The model under review builds one solid part; all positions refer to its coordinate system, in mm. Face numbers are marked on the shaded views. A direction names the side the tool comes from. Give positions to 0.01 mm unless a question says otherwise; leave off trailing zeros. Loops run counter-clockwise (first coordinate to the right, second up) from the corner with the lowest first, then second, coordinate; pieces in that order, holes last. Notation, with made-up numbers: M -14.5,7 L 42.5,7 A20 ccw 42.5,32 Z; hole C 58.25,80 d10. An arc over 180 degrees is marked long. Return JSON: item names as keys, results as strings.
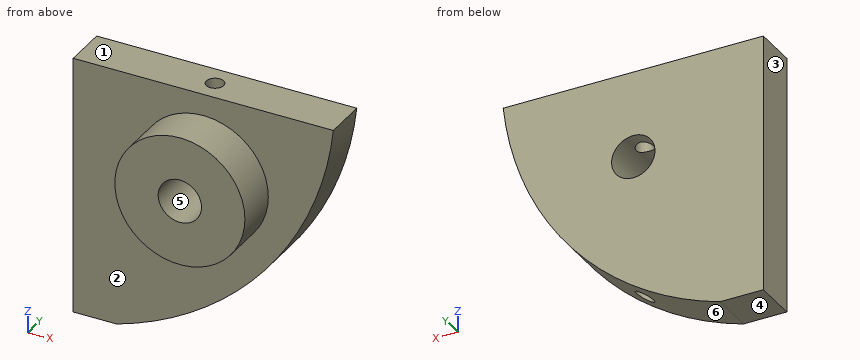
```python
from build123d import *

# Parameters (mm, degrees)
F1_DEPTH = 6.35
F2_R     = 19.05
F3_DEPTH = 12.7
F4_R     = 6.35
F5_DEPTH = 74.422
F6_R     = 2.54
F7_DEPTH = 76.201


with BuildPart() as f1:
    # F0 (on Front) → F1 (new body, symmetric)
    with BuildSketch(Plane.XZ):
        with BuildLine():
            Line((2.516038, 58.73151), (-73.683962, 58.73151))
            Line((-73.683962, 58.73151), (-73.683962, -17.46849))
            Line((-73.683962, -17.46849), (-60.983962, -17.46849))
            ThreePointArc((-60.983962, -17.46849), (-17.618712, 10.952135), (2.516038, 58.73151))
        make_face()
    extrude(amount=F1_DEPTH, both=True)

    # F2 (on face) → F3 (join)
    with BuildSketch(Plane.XZ.offset(6.35)):
        with Locations((-35.583962, 33.33151)):
            Circle(F2_R)
    extrude(amount=F3_DEPTH)

    # F4 (on face) → F5 (cut)
    with BuildSketch(Plane.XZ.offset(19.05)):
        with Locations((-35.583962, 33.33151)):
            Circle(F4_R)
    extrude(amount=-F5_DEPTH, mode=Mode.SUBTRACT)

    # F6 (on face) → F7 (cut, through all)
    with BuildSketch(Plane.XY.offset(58.73151)):
        with Locations((-35.583962, 0)):
            Circle(F6_R)
    extrude(amount=-F7_DEPTH, mode=Mode.SUBTRACT)


solid = f1.part
```
1) Consider section C-C on x = -50.5. Write out the cut boundary in (y, z), then the cut area to 3 significant figures.
From the geometry:
{"outline": "M -19.05,21.48 L -6.35,21.48 L -6.35,-13.68 L 6.35,-13.68 L 6.35,58.73 L -6.35,58.73 L -6.35,45.18 L -19.05,45.18 Z", "area": "1,220 mm²"}
2) Insertion check: pin 1 (6.5 mm diameter, centred on x = -35.58, y = 0, fed in from -Z); pin 2 (8 mm diameter, centred on x = -35.58, y = 0, fed in from -Z); pin 3 (8 mm diameter, centred on y = 2.5, z = 16, fed in from +X); pin 4 (4 mm diameter, centred on y = -7.5, z = 16, fed in from -X). Each pin has a flat end and moves straight along its axis. Give the tip position at first contact, or say it passes through.
From the geometry:
{"pin 1": "z = -7.54", "pin 2": "z = -8.01", "pin 3": "x = -11", "pin 4": "x = -73.68"}
3) Wall thickness on L1, parallel to Y at x = -63.5, z = 25; L2, parallel to X at y = 0, z = 19; L3, parallel to X at y = 0, z = 16: over which ranges is each line inside the solid? List them lowest first. Write a range as from..to.
From the geometry:
{"L1": "-6.35..6.35", "L2": "-73.68..-38.12, -33.04..-11.65", "L3": "-73.68..-38.12, -33.04..-13.71"}
4) Consider section B-B on z = 22. Write out the cut boundary in (x, y).
From the geometry:
{"outline": "M -73.68,-6.35 L -50.9,-6.35 L -50.9,-19.05 L -20.27,-19.05 L -20.27,-6.35 L -9.76,-6.35 L -9.76,6.35 L -73.68,6.35 Z; hole C -35.58,0 d5.08"}
5) Consider section A-A on y = 0. Write out the cut boundary in (x, z), then the cut area to 3 significant figures.
From the geometry:
{"outline": "M -73.68,-17.47 L -60.98,-17.47 A88.9 ccw -38.12,-7.1 L -38.12,27.51 A6.35 cw -38.12,39.15 L -38.12,58.73 L -73.68,58.73 Z; M -33.04,-3.61 A88.9 ccw 2.52,58.73 L -33.04,58.73 L -33.04,39.15 A6.35 cw -33.04,27.51 Z", "area": "4,020 mm²"}
6) Tool access review of the marked faces 1 and 2: name each direction out of +Z, -Z, +X, -X, +Y, -Y from which nothing blocks a thin tool from reaching the whole face with its end or side.
From the geometry:
{"face 1": "+Z, +X, -X, +Y, -Y", "face 2": "-Y"}
7) Consider section D-D on z = -6. Write out the cut boundary in (x, y), then the cut area to 3 significant figures.
From the geometry:
{"outline": "M -73.68,-6.35 L -36.44,-6.35 L -36.44,-2.39 A2.54 cw -36.44,2.39 L -36.44,6.35 L -73.68,6.35 Z", "area": "467 mm²"}
8) The part is to be moulded in two halves that separate along X. For the marked faces 3, 4, 5 and 6, say which applies: released by +X, released by -X, zero draft, split by the parting line, or undercut.
From the geometry:
{"face 3": "released by -X", "face 4": "zero draft", "face 5": "undercut", "face 6": "released by +X"}
